Part model, mm, in its own coordinate system. Face numbers are marked on the shaded views. A direction names the side the tool comes from. Coordinates: 2 decimals unless noted, no trailing zeros. Loops run counter-clockwise (first coordinate to the right, second up) from the corner with the lowest first, then second, coordinate; pieces in that order, holes last. Notation, with made-up numbers: (46.5, 17.5) - (99.5, 17.5) arc R25 cw to (99.5, 48.5) - close; hole circle Ø1 at (6.25, -14). An arc over 180 degrees is marked (long way). Answer as CSV lines item,"result".
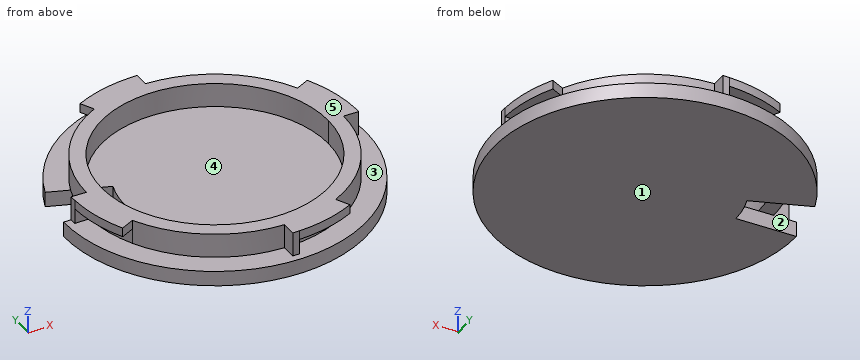
from build123d import *

# Parameters (mm, degrees)
F1_DEPTH = 8
F2_DEPTH = 8
F3_START = 5
F3_DEPTH = 3
F4_R     = 50
F5_DEPTH = 5
F7_DEPTH = 5


with BuildPart() as f1:
    # F0 (on Top) → F1 (new body)
    with BuildSketch(Plane.XY):
        with BuildLine():
            ThreePointArc((19.4384842845, -37.7941176471), (36.2793714257, -22.137235802), (42.5, 0))
            ThreePointArc((42.5, 0), (42.488227143, 1.0002770852), (42.4529150943, 2))
            ThreePointArc((42.4529150943, 2), (41.0599774657, 10.969423436), (37.7941176471, 19.4384842845))
            ThreePointArc((37.7941176471, 19.4384842845), (22.137235802, 36.2793714257), (0, 42.5))
            ThreePointArc((0, 42.5), (-1.0002770852, 42.488227143), (-2, 42.4529150943))
            ThreePointArc((-2, 42.4529150943), (-10.969423436, 41.0599774657), (-19.4384842845, 37.7941176471))
            ThreePointArc((-19.4384842845, 37.7941176471), (-36.2793714257, 22.137235802), (-42.5, 0))
            ThreePointArc((-42.5, 0), (-42.488227143, -1.0002770852), (-42.4529150943, -2))
            ThreePointArc((-42.4529150943, -2), (-41.0599774657, -10.969423436), (-37.7941176471, -19.4384842845))
            ThreePointArc((-37.7941176471, -19.4384842845), (-22.137235802, -36.2793714257), (0, -42.5))
            ThreePointArc((0, -42.5), (1.0002770852, -42.488227143), (2, -42.4529150943))
            ThreePointArc((2, -42.4529150943), (10.969423436, -41.0599774657), (19.4384842845, -37.7941176471))
        make_face()
        with BuildLine():
            ThreePointArc((37.5, 0), (8.8235294118, -36.4471580335), (-33.3477508651, -17.1516037805))
            ThreePointArc((-33.3477508651, -17.1516037805), (-8.8235294118, 36.4471580335), (37.5, 0))
        make_face(mode=Mode.SUBTRACT)
    extrude(amount=F1_DEPTH)

    # F0 (on Top) → F2 (join)
    with BuildSketch(Plane.XY):
        with BuildLine():
            ThreePointArc((-47.5, 0), (-47.486842101, -1.1179567422), (-47.4473756936, -2.2352941176))
            Line((-47.4473756936, -2.2352941176), (-42.4529150943, -2))
            ThreePointArc((-42.4529150943, -2), (-42.488227143, -1.0002770852), (-42.5, 0))
            Line((-42.5, 0), (-47.5, 0))
        make_face()
        with BuildLine():
            Line((0, 42.5), (0, 47.5))
            ThreePointArc((0, 47.5), (-1.1179567422, 47.486842101), (-2.2352941176, 47.4473756936))
            Line((-2.2352941176, 47.4473756936), (-2, 42.4529150943))
            ThreePointArc((-2, 42.4529150943), (-1.0002770852, 42.488227143), (0, 42.5))
        make_face()
        with BuildLine():
            Line((42.5, 0), (47.5, 0))
            ThreePointArc((47.5, 0), (47.486842101, 1.1179567422), (47.4473756936, 2.2352941176))
            Line((47.4473756936, 2.2352941176), (42.4529150943, 2))
            ThreePointArc((42.4529150943, 2), (42.488227143, 1.0002770852), (42.5, 0))
        make_face()
        with BuildLine():
            ThreePointArc((0, -47.5), (1.1179567422, -47.486842101), (2.2352941176, -47.4473756936))
            Line((2.2352941176, -47.4473756936), (2, -42.4529150943))
            ThreePointArc((2, -42.4529150943), (1.0002770852, -42.488227143), (0, -42.5))
            Line((0, -42.5), (0, -47.5))
        make_face()
    extrude(amount=F2_DEPTH)

    # F0 (on Top) → F3 (join)
    with BuildSketch(Plane.XY.offset(F3_START)):
        with BuildLine():
            ThreePointArc((-47.4473756936, -2.2352941176), (-45.8905630499, -12.2599438402), (-42.2404844291, -21.7253647886))
            Line((-42.2404844291, -21.7253647886), (-37.7941176471, -19.4384842845))
            ThreePointArc((-37.7941176471, -19.4384842845), (-41.0599774657, -10.969423436), (-42.4529150943, -2))
            Line((-42.4529150943, -2), (-47.4473756936, -2.2352941176))
        make_face()
        with BuildLine():
            ThreePointArc((2.2352941176, -47.4473756936), (12.2599438402, -45.8905630499), (21.7253647886, -42.2404844291))
            Line((21.7253647886, -42.2404844291), (19.4384842845, -37.7941176471))
            ThreePointArc((19.4384842845, -37.7941176471), (10.969423436, -41.0599774657), (2, -42.4529150943))
            Line((2, -42.4529150943), (2.2352941176, -47.4473756936))
        make_face()
        with BuildLine():
            Line((42.4529150943, 2), (47.4473756936, 2.2352941176))
            ThreePointArc((47.4473756936, 2.2352941176), (45.8905630499, 12.2599438402), (42.2404844291, 21.7253647886))
            Line((42.2404844291, 21.7253647886), (37.7941176471, 19.4384842845))
            ThreePointArc((37.7941176471, 19.4384842845), (41.0599774657, 10.969423436), (42.4529150943, 2))
        make_face()
        with BuildLine():
            Line((-2, 42.4529150943), (-2.2352941176, 47.4473756936))
            ThreePointArc((-2.2352941176, 47.4473756936), (-12.2599438402, 45.8905630499), (-21.7253647886, 42.2404844291))
            Line((-21.7253647886, 42.2404844291), (-19.4384842845, 37.7941176471))
            ThreePointArc((-19.4384842845, 37.7941176471), (-10.969423436, 41.0599774657), (-2, 42.4529150943))
        make_face()
    extrude(amount=F3_DEPTH)

    # F4 (on Top) → F5 (join)
    with BuildSketch(Plane.XY):
        Circle(F4_R)
    extrude(amount=-F5_DEPTH)

    # F6 (on Top) → F7 (cut)
    with BuildSketch(Plane.XY):
        with BuildLine():
            Line((-28.3333333333, 9.8601329718), (-47.2222222222, 16.4335549531))
            ThreePointArc((-47.2222222222, 16.4335549531), (-49.3006648592, 8.3333333333), (-50, 0))
            Line((-50, 0), (-30, 0))
            ThreePointArc((-30, 0), (-29.5803989155, 5), (-28.3333333333, 9.8601329718))
        make_face()
    extrude(amount=-F7_DEPTH, mode=Mode.SUBTRACT)


solid = f1.part
Q1. Flat gauge pins, fed straight in: pin 1 (5 mm diameter, centred on y = -29.5, z = 4, fed in from -X); pin 2 (4 mm diameter, centred on y = 45, z = 3, fed in from +X); pin 3 (4 mm diameter, centred on x = 9, z = -3.5, fed in from +Y). Where does each tip first touch, or does it go through?
Results:
pin 1,"stops at x = -32.82"
pin 2,"stops at x = 0"
pin 3,"stops at y = 49.51"
Q2. Saw through at B-B (y = -13). Give the cut face in (x, z), then the cut area to 3 significant figures.
Results:
outline,"(-48.28, -5) - (48.28, -5) - (48.28, 0) - (40.46, 0) - (40.46, 8) - (35.17, 8) - (35.17, 0) - (-35.17, 0) - (-35.17, 8) - (-45.69, 8) - (-45.69, 5) - (-40.46, 5) - (-40.46, 0) - (-48.28, 0) - close"
area,"583 mm^2"
Q3. Which spindle directions (+Z, -Z, +X, -X, +Y, -Y) get a long thin tool onto all of the face, cutting with end or side? Do the marked faces 1, 2 and 3. Say none if no direction does.
Results:
face 1,"-Z, +X, -X, +Y, -Y"
face 2,"-Z, -X"
face 3,"none"
Q4. Wall check: L1, parallel to X at y = -0.5, z = 1.75; L2, parallel to X at y = 21, z = 7.25; L3, parallel to Z at x = 0, y = -5. Give the ranges that are in metal, low to high.
Results:
L1,"x = -47.5 to -37.5, 37.5 to 42.5"
L2,"x = -36.95 to -31.07, 31.07 to 36.95, 40.83 to 42.61"
L3,"z = -5 to 0"
Q5. Saw through at A-A (z = 1.75). Give the cut face in (x, y), then the cut area to 3 significant figures.
Results:
outline,"(-47.5, 0) arc R47.5 ccw to (-47.45, -2.24) - (-42.45, -2) arc R42.5 ccw to (0, -42.5) - (0, -47.5) arc R47.5 ccw to (2.24, -47.45) - (2, -42.45) arc R42.5 ccw to (42.5, 0) - (47.5, 0) arc R47.5 ccw to (47.45, 2.24) - (42.45, 2) arc R42.5 ccw to (0, 42.5) - (0, 47.5) arc R47.5 ccw to (-2.24, 47.45) - (-2, 42.45) arc R42.5 ccw to (-42.5, 0) - close; hole circle Ø75 at (0, 0)"
area,"1,300 mm^2"
Q6. Saw through at D-D (y = -31.5). Give the cut face in (x, z), then the cut area to 3 significant figures.
Results:
outline,"(-38.83, -5) - (38.83, -5) - (38.83, 0) - (28.53, 0) - (28.53, 8) - (20.35, 8) - (20.35, 0) - (-20.35, 0) - (-20.35, 8) - (-28.53, 8) - (-28.53, 0) - (-38.83, 0) - close"
area,"519 mm^2"
Q7. Two-plate mould, pull along Y, no slides. Class the marked faces 4 and 5: released by +Y, released by -Y, zero draft, split by the parting line, or undercut.
Results:
face 4,"undercut"
face 5,"zero draft"
Q8. Saw through at C-C (x = -26). Give the cut face in (y, z).
Results:
outline,"(-42.71, -5) - (42.71, -5) - (42.71, 0) - (33.62, 0) - (33.62, 8) - (27.02, 8) - (27.02, 0) - (-27.02, 0) - (-27.02, 8) - (-33.62, 8) - (-33.62, 0) - (-42.71, 0) - close"
